Verification items for the finished model (mm, model axes). Give positions to 0.01 mm unless a question says otherwise; leave off trailing zeros. Order: outer loops, then holes, each group sorted by start corner. A loop starts at its lowest first (then second) coordinate and runs counter-clockwise, first axis right, second up.
from build123d import *

# Parameters (mm, degrees)
F0_R     = 185
F1_DEPTH = 900
F4_DEPTH = 200
F5_R     = 110
F5_R_2   = 7
F6_DEPTH = 25
F7_R     = 8


with BuildPart() as f1:
    # F0 (on Top) → F1 (new body)
    with BuildSketch(Plane.XY):
        Circle(F0_R)
    extrude(amount=F1_DEPTH)

    # F3 (on face) → F4 (join)
    with BuildSketch(Plane.XY.offset(900)):
        with BuildLine():
            ThreePointArc((83.400185, -26.469967), (75.780776, -30.745971), (78.266953, -39.122041))
            ThreePointArc((78.266953, -39.122041), (81.080729, -32.896282), (83.400185, -26.469967))
        make_face()
        with BuildLine():
            ThreePointArc((83.400185, -26.469967), (81.080729, -32.896282), (78.266953, -39.122041))
            ThreePointArc((78.266953, -39.122041), (85.507452, -39.58259), (89.267234, -33.377674))
            ThreePointArc((89.267234, -33.377674), (87.602525, -28.846154), (83.400185, -26.469967))
        make_face()
        with BuildLine():
            ThreePointArc((-68.096127, -54.946951), (-72.208025, -49.419138), (-75.872273, -43.584954))
            ThreePointArc((-75.872273, -43.584954), (-78.807669, -53.935931), (-68.096127, -54.946951))
        make_face()
        with BuildLine():
            ThreePointArc((-68.096127, -54.946951), (-66.56789, -52.670867), (-66.031027, -49.9824))
            ThreePointArc((-66.031027, -49.9824), (-69.215842, -44.113469), (-75.872273, -43.584954))
            ThreePointArc((-75.872273, -43.584954), (-72.208025, -49.419138), (-68.096127, -54.946951))
        make_face()
        with BuildLine():
            ThreePointArc((-4.602196, 87.378886), (-11.519275, 86.738436), (-18.36375, 85.551287))
            ThreePointArc((-18.36375, 85.551287), (-11.355664, 78.567501), (-4.363768, 85.567496))
            ThreePointArc((-4.363768, 85.567496), (-4.423631, 86.481003), (-4.602196, 87.378886))
        make_face()
        with BuildLine():
            ThreePointArc((-4.602196, 87.378886), (-12.28531, 92.506571), (-18.36375, 85.551287))
            ThreePointArc((-18.36375, 85.551287), (-11.519275, 86.738436), (-4.602196, 87.378886))
        make_face()
    extrude(amount=F4_DEPTH)

    # F5 (on face) → F6 (join)
    with BuildSketch(Plane.XY.offset(1100)):
        Circle(F5_R)
        with Locations((-11.363768, 85.567496)):
            Circle(F5_R_2, mode=Mode.SUBTRACT)
        with Locations((-11.363768, 85.567496)):
            Circle(F5_R_2)
    extrude(amount=F6_DEPTH)

    # F7
    f7_edges = [f1.edges().sort_by_distance(p)[0] for p in [
        (-110, 0, 1100),
    ]]
    fillet(f7_edges, radius=F7_R)


solid = f1.part
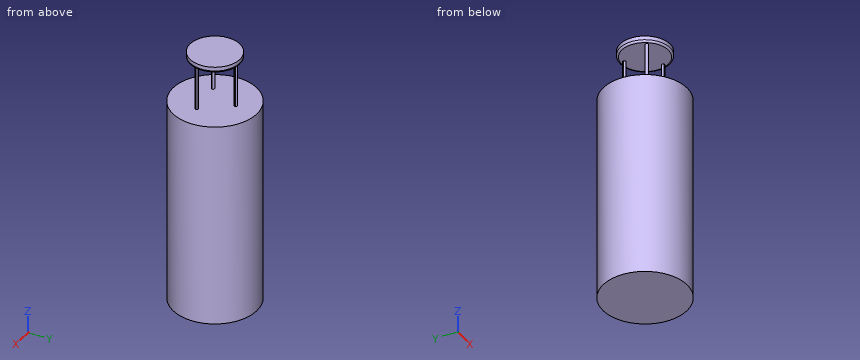
(1) Section check D-D, the plane y = -130. Enter the section's corners in (x, z), then the cut area to 3 significant figures.
Solved:
outline: (-131.62, 0) - (131.62, 0) - (131.62, 900) - (-131.62, 900) - close
area: 237,000 mm2
(2) Section check B-B, the plane z = 773.5. Enter the section's corners in (x, y).
Solved:
outline: circle Ø370 at (0, 0)
(3) Section check A-A, the plane y = 0. Enter the section's corners in (x, z), then the cut area to 3 significant figures.
Solved:
outline: (-185, 0) - (185, 0) - (185, 900) - (-185, 900) - close; (-110, 1108) arc R8 ccw to (-102, 1100) - (102, 1100) arc R8 ccw to (110, 1108) - (110, 1125) - (-110, 1125) - close
area: 338,000 mm2
(4) Go/stop test with flat-tipped pins: pin 1 (10 mm diameter, centred on x = 115, z = 894.5, fed in from +Y); pin 2 (8 mm diameter, centred on y = -78, z = 826.5, fed in from +X); pin 3 (4 mm diameter, centred on y = -40, z = 493, fed in from +X). Record where each tip stops, or that it passes through.
Solved:
pin 1: stops at y = 148.74
pin 2: stops at x = 169.56
pin 3: stops at x = 181.06
(5) Section check C-C, the plane x = 153.5. Enter the section's corners in (y, z), then the cut area to 3 significant figures.
Solved:
outline: (-103.26, 0) - (103.26, 0) - (103.26, 900) - (-103.26, 900) - close
area: 186,000 mm2
(6) Scan lines: line 1 (Z direction, x = -135, y = 37.5); line 2 (Z direction, x = 71, y = -64); line 3 (X direction, y = -8, z = 655.5). Record each from-to range of solid material in increasing order.
Solved:
line 1: z = 0 to 900
line 2: z = 0 to 900, 1100 to 1125
line 3: x = -184.83 to 184.83
